Read the model definition and answer for the solid it produces. Units are mm, in the model's axes. Face numbers are marked on the shaded views. A direction names the side the tool comes from. Give positions to 0.01 mm unless a question says otherwise; leave off trailing zeros. Write each loop counter-clockwise with the first axis right and the second up, starting at its lowest first coordinate (ties: lowest second). Pieces come first, ordered by that corner, then holes.
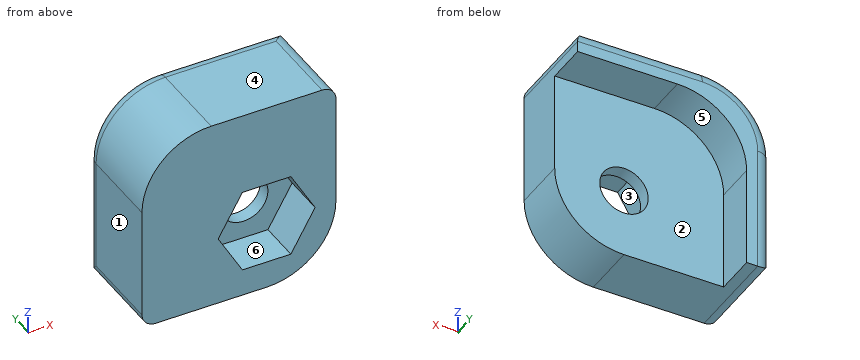
Autodesk Inventor part; units mm, degrees
ref_plane "YZ Plane" through (0, 0, 0) normal (1, 0, 0) x (0, 1, 0)
ref_plane "XZ Plane" through (0, 0, 0) normal (0, 1, 0) x (-1, 0, 0)
ref_plane "XY Plane" through (0, 0, 0) normal (0, 0, 1) x (1, 0, 0)
sketch "Sketch1" plane through (0, 0, 0) normal (0, 1, 0) x (-1, 0, 0)
  line L0 (0, 0) -> (14, 0)
  line L1 (14, 0) -> (14, 14)
  line L2 (14, 14) -> (0, 14)
  line L3 (0, 14) -> (0, 0)
  circle A0 centre (5, 5) radius 1.75
  line L4 (0, 0) -> (12.2, 0)
  line L5 (12.2, 0) -> (12.2, 12.2)
  line L6 (12.2, 12.2) -> (0, 12.2)
  line L7 (0, 12.2) -> (0, 0)
  circle A1 centre (5, 5) radius 3.5
  line L8 (1.5, 5) -> (3.25, 8.0311)
  line L9 (3.25, 8.0311) -> (6.75, 8.0311)
  line L10 (6.75, 8.0311) -> (8.5, 5)
  line L11 (8.5, 5) -> (6.75, 1.9689)
  line L12 (6.75, 1.9689) -> (3.25, 1.9689)
  line L13 (3.25, 1.9689) -> (1.5, 5)
  dimension "d19" = 7
  dimension "d0" = 14
  dimension "d1" = 14
  dimension "d2" = 3.5
  dimension "d3" = 5
  dimension "d4" = 5
  dimension "d5" = 12.2
  dimension "d6" = 12.2
extrude "Extrusion3" add sketch "Sketch1" along normal blind 4 contours L3 L6 L5 L0 | L10 A1 | L11 L12 L13 L8 L9 L10 | A1 L11 | L9 A1 | A1 L12 | L8 A1 | A1 L13
extrude "Extrusion4" add sketch "Sketch1" along normal blind 7 contours L5 L6 L3 L2 L1 L0
fillet "Fillet3" radius 5 3 edges at (0, 2, 0) (-12.2, 5.5, 12.2) (-14, 3.5, 14)
fillet "Fillet4" radius 1 5 edges at (-12.5355, 7, 12.5355) (-4.5, 7, 14) (-14, 7, 4.5) (-14, 3.5, 0) (0, 3.5, 14)
extrude "Extrusion5" cut sketch "Sketch1" along normal blind 3 contours L11 L12 L13 L8 L9 L10
properties part number "RxBoardMountFootWithNut"
Item 1: Section D-D (y = 5.75) is taken. Write down the section's boundary in (x, z), and give its area (3 significant figures).
Result set:
outline: (-14, 1) arc R1 ccw to (-13, 0) - (-12.2, 0) - (-12.2, 7.2) arc R5 cw to (-7.2, 12.2) - (0, 12.2) - (0, 13) arc R1 ccw to (-1, 14) - (-9, 14) arc R5 ccw to (-14, 9) - close
area: 46.7 mm2
Item 2: Section A-A (y = 1.75) is taken. Write down the section's boundary in (x, z).
Result set:
outline: (-14, 1) arc R1 ccw to (-13, 0) - (-5, 0) arc R5 ccw to (0, 5) - (0, 13) arc R1 ccw to (-1, 14) - (-9, 14) arc R5 ccw to (-14, 9) - close; hole (-8.5, 5) - (-6.75, 1.97) - (-3.25, 1.97) - (-1.5, 5) - (-3.25, 8.03) - (-6.75, 8.03) - close
Item 3: Each of these flat-tipped pins is pushed along its axis until it touches: pin 1 Ø4 at (x, z) = (-5, 5) entering from +Y; pin 2 Ø1.5 at (x, y) = (-2, 6) entering from -Z; pin 3 Ø1.5 at (y, z) = (5.5, 4) entering from +X; pin 4 Ø3.5 at (x, y) = (-5, 1) entering from -Z. Where does it stop, or does it pass through?
Result set:
pin 1: stops at y = 4
pin 2: stops at z = 12.2
pin 3: stops at x = -12.2
pin 4: stops at z = 0
Item 4: Which of the six approach directions +Z, -Z, +X, -X, +Y, -Y give full straight-line access (tool end or side, diameter ignored) to the marked faces 4, 5 and 6?
Result set:
face 4: +Z, +X, -X, +Y, -Y
face 5: -Z, +X, +Y
face 6: -Y
Item 5: Find the intervals of material crossed by line 1 along Z through (x, y) = (-5, 3.45); line 2 along Y through (x, z) = (-8.75, 1.75); line 3 along Z through (x, y) = (-1.25, 4.75), in increasing order.
Result set:
line 1: z = 0 to 3.25, 6.75 to 14
line 2: y = 0 to 4
line 3: z = 12.2 to 14
Item 6: Section C-C (z = 6.5) is taken. Write down the section's boundary in (x, y).
Result set:
outline: (-14, 0) - (-7.63, 0) - (-7.63, 3) - (-5.9, 3) - (-5.9, 4) - (-12.2, 4) - (-12.2, 7) - (-13, 7) arc R1 ccw to (-14, 6) - close; (-4.1, 3) - (-2.37, 3) - (-2.37, 0) - (0, 0) - (0, 4) - (-4.1, 4) - close
Item 7: Determine the mould class of the marked faces 1, 2 and 3 for opening direction X: pulls with the +X half, pulls with the -X half, needs draft (parallel to the pull), parting line crosses it, or undercut.
Result set:
face 1: pulls with the -X half
face 2: needs draft
face 3: undercut
Item 8: Section B-B (x = -4.75) is taken. Write down the section's boundary in (y, z), and give its area (3 significant figures).
Result set:
outline: (0, 0.01) - (4, 0.01) - (4, 3.27) - (3, 3.27) - (3, 1.97) - (0, 1.97) - close; (0, 8.03) - (3, 8.03) - (3, 6.73) - (4, 6.73) - (4, 12.2) - (7, 12.2) - (7, 13) arc R1 ccw to (6, 14) - (0, 14) - close
area: 39.5 mm2
